Verification items for the finished model (mm, model axes). A direction names the side the tool comes from. Coordinates: 2 decimals unless noted, no trailing zeros. Order: outer loops, then holes, each group sorted by start corner. A loop starts at its lowest first (then second) coordinate and runs counter-clockwise, first axis right, second up. Notation, with made-up numbers: M 61.25,58 L 74.25,58 A7 ccw 74.25,71 Z; hole C -8,21 d11. An arc over 180 degrees is marked long. Return JSON: item names as keys, results as strings.
```python
from build123d import *

# Parameters (mm, degrees)
F1_DEPTH = 15
F2_R     = 10
F3_DEPTH = 5


with BuildPart() as f1:
    # F0 (on Top) → F1 (new body)
    with BuildSketch(Plane.XY):
        Polygon((-12.7223648903, -0.643178855), (-5.8452739672, 11.2682920321), (-19.6474669216, 11.1839482352), align=None)
        Polygon((0.0316754732, 11.3042054723), (-5.8452739672, 11.2682920321), (-12.7223648903, -0.643178855), (-6.8359901735, -10.6963017637), (0.1007524936, -10.6963017637), align=None)
        Polygon((0.0316754732, 11.3042054723), (0, 21.3926035274), (-5.8452739672, 11.2682920321), align=None)
        Polygon((5.8041732175, 11.3394806187), (0, 21.3926035274), (0.0316754732, 11.3042054723), align=None)
        Polygon((12.6812641407, -0.5719902684), (5.8041732175, 11.3394806187), (0.0316754732, 11.3042054723), (0.1007524936, -10.6963017637), (6.9181916728, -10.6963017637), align=None)
        Polygon((19.509316747, 11.4232313565), (5.8041732175, 11.3394806187), (12.6812641407, -0.5719902684), align=None)
        Polygon((18.5265381078, -10.6963017637), (12.6812641407, -0.5719902684), (6.9181916728, -10.6963017637), align=None)
        Polygon((0.1381501745, -22.6071795917), (0.1007524936, -10.6963017637), (-6.8359901735, -10.6963017637), align=None)
        Polygon((6.9181916728, -10.6963017637), (0.1007524936, -10.6963017637), (0.1381501745, -22.6071795917), align=None)
        Polygon((-6.8359901735, -10.6963017637), (-12.7223648903, -0.643178855), (-18.5265381078, -10.6963017637), align=None)
    extrude(amount=F1_DEPTH)

    # F2 (on face) → F3 (join)
    with BuildSketch(Plane.XY.offset(15)):
        Polygon((-5.8452739672, 11.2682920321), (-19.6474669216, 11.1839482352), (-12.7223648903, -0.643178855), (-18.5265381078, -10.6963017637), (-6.8359901735, -10.6963017637), (0.1381501745, -22.6071795917), (6.9181916728, -10.6963017637), (18.5265381078, -10.6963017637), (12.6812641407, -0.5719902684), (19.509316747, 11.4232313565), (5.8041732175, 11.3394806187), (0, 21.3926035274), align=None)
        Circle(F2_R, mode=Mode.SUBTRACT)
    extrude(amount=F3_DEPTH)


solid = f1.part
```
Q1. Material ranges on line 1 along X through (y, z) = (-1, 19.25); line 2 along Z through (x, y) = (2, -2); line 3 along X through (y, z) = (-12, 15.5), recorded low to high.
Values:
{"line 1": "-12.93 to -9.95, 9.95 to 12.93", "line 2": "0 to 15", "line 3": "-6.07 to 6.18"}
Q2. Tool access check on faces 4 (the face through (13, -10.696, 10)), 5 (the face through (16.047, 5.342, 9.86)), 6 (the face through (0, 0, 15)), 7 (the face through (-15.584, -5.599, 9.86)). Record the directions out of +Z, -Z, +X, -X, +Y, -Y that give a thin tool (end or side, any length) a straight path to the whole face; none if there is none.
Values:
{"face 4": "+Z, -Z, +X, -Y", "face 5": "+Z, -Z, +X", "face 6": "+Z", "face 7": "+Z, -Z, -X"}
Q3. Cross-section at B-B, the plane z = 7.75. Record the boundary of the cut face in (x, y), and give its area (3 significant figures).
Values:
{"outline": "M -19.65,11.18 L -12.72,-0.64 L -18.53,-10.7 L -6.84,-10.7 L 0.14,-22.61 L 6.92,-10.7 L 18.53,-10.7 L 12.68,-0.57 L 19.51,11.42 L 5.8,11.34 L 0,21.39 L -5.85,11.27 Z", "area": "840 mm^2"}
Q4. Cross-section at D-D, the plane y = 0. Record the boundary of the cut face in (x, z).
Values:
{"outline": "M -13.1,0 L 13.01,0 L 13.01,20 L 10,20 L 10,15 L -10,15 L -10,20 L -13.1,20 Z"}
Q5. Cross-section at C-C, the plane x = -8.5. Record the boundary of the cut face in (y, z), and give its area (3 significant figures).
Values:
{"outline": "M -10.7,0 L 11.25,0 L 11.25,20 L 5.27,20 L 5.27,15 L -5.27,15 L -5.27,20 L -10.7,20 Z", "area": "386 mm^2"}
Q6. Go/stop test with flat-tipped pins: pin 1 (8 mm diameter, centred on x = 9, z = 9.5, fed in from +Y); pin 2 (2 mm diameter, centred on x = -5, z = 5.5, fed in from +Y); pin 3 (6 mm diameter, centred on x = 11, z = 14, fed in from -Y). Record where each tip stops, or that it passes through.
Values:
{"pin 1": "y = 12.73", "pin 2": "y = 14.46", "pin 3": "y = -10.7"}
Q7. Cross-section at A-A, the plane x = 13.5. Record the boundary of the cut face in (y, z), and give its area (3 significant figures).
Values:
{"outline": "M -10.7,0 L -1.99,0 L -1.99,20 L -10.7,20 Z; M 0.87,0 L 11.39,0 L 11.39,20 L 0.87,20 Z", "area": "385 mm^2"}
Q8. Draft check along X on faces 1 (the face through (15.645, -5.705, 9.86)), 2 (the face through (-2.17, -9.76, 17.46)), 3 (the face through (-13, -10.696, 10)). Enter one of: pulls with the +X half, pulls with the -X half, needs draft (parallel to the pull), parting line crosses it, or undercut.
Values:
{"face 1": "pulls with the +X half", "face 2": "undercut", "face 3": "needs draft"}
